Verification items for the finished model (mm, model axes). Face numbers are marked on the shaded views. Give positions to 0.01 mm unless a question says otherwise; leave off trailing zeros. Loops run counter-clockwise (first coordinate to the right, second up) from the corner with the lowest first, then second, coordinate; pieces in that order, holes last. Notation, with made-up numbers: M -15.75,-13 L -7.75,-13 A17 cw -7.75,0 Z; hole C 36.5,58.5 d5. An arc over 180 degrees is marked long. Answer in a Markdown table with one row per item.
Autodesk Inventor part; units mm, degrees
ref_plane "YZ Plane" through (0, 0, 0) normal (1, 0, 0) x (0, 1, 0)
ref_plane "XZ Plane" through (0, 0, 0) normal (0, 1, 0) x (-1, 0, 0)
ref_plane "XY Plane" through (0, 0, 0) normal (0, 0, 1) x (1, 0, 0)
sketch "Sketch1" plane through (0, 0, 0) normal (0, 0, 1) x (1, 0, 0)
  circle A0 centre (0, 0) radius 5
  line L0 (-15, -20) -> (15, -20)
  line L1 (15, -20) -> (15, 20)
  line L2 (15, 20) -> (-15, 20)
  line L3 (-15, 20) -> (-15, -20)
  line L4 (-15, -20) -> (15, 20) construction
  line L5 (15, -20) -> (-15, 20) construction
  dimension "d0" = 10
  dimension "d1" = 30
  dimension "d2" = 40
extrude "Extrusion1" add sketch "Sketch1" along normal mid plane 10
properties part number "Corredera" material "Stainless Steel"
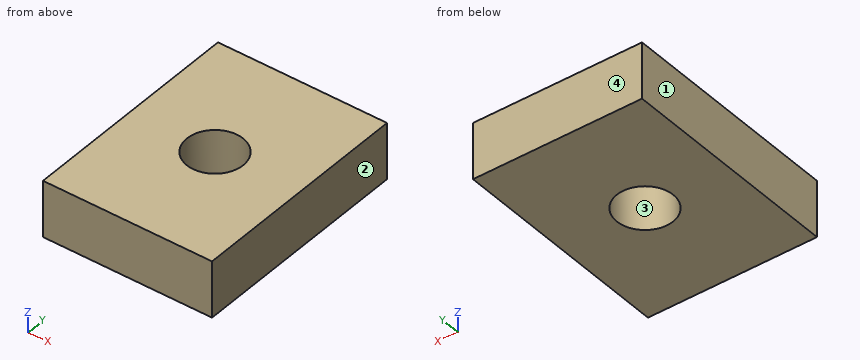
Item 1: Sectioned sample at B-B (x = 0). Record the cut outline in (y, z).
Reported:
| item | result |
|---|---|
| outline | M -20,-5 L -5,-5 L -5,5 L -20,5 Z; M 5,-5 L 20,-5 L 20,5 L 5,5 Z |
Item 2: Scan lines: L1, parallel to Y at x = 0, z = 1; L2, parallel to Y at x = -4, z = 1.5; L3, parallel to X at y = -4, z = -2. Record each from-to range of solid material in increasing order. Write a range as [from, to].
Reported:
| item | result |
|---|---|
| L1 | y = [-20, -5], [5, 20] |
| L2 | y = [-20, -3], [3, 20] |
| L3 | x = [-15, -3], [3, 15] |
Item 3: Release check for a two-part mould opening along X. For the marked faces 1, 2, 3 and 4 record: released by +X, released by -X, zero draft, split by the parting line, or undercut.
Reported:
| item | result |
|---|---|
| face 1 | released by -X |
| face 2 | released by +X |
| face 3 | undercut |
| face 4 | zero draft |
Item 4: Go/stop test with a flat-tipped pin: pin 1 (8 mm diameter, centred on x = 0, y = 0, fed in from +Z). Record where the tip stops, or that it passes through.
Reported:
| item | result |
|---|---|
| pin 1 | passes through |
Item 5: Sectioned sample at C-C (z = 4.25). Record the cut outline in (x, y).
Reported:
| item | result |
|---|---|
| outline | M -15,-20 L 15,-20 L 15,20 L -15,20 Z; hole C 0,0 d10 |
Item 6: Sectioned sample at A-A (y = 0). Record the cut outline in (x, z), and give its area (3 significant figures).
Reported:
| item | result |
|---|---|
| outline | M -15,-5 L -5,-5 L -5,5 L -15,5 Z; M 5,-5 L 15,-5 L 15,5 L 5,5 Z |
| area | 200 mm^2 |
